from build123d import *

# Parameters (mm, degrees)
SKETCH1_W           = 8
SKETCH1_H           = 16
SKETCH1_R           = 1.55
BOSS_EXTRUDE1_DEPTH = 6
CUT_EXTRUDE1_DEPTH  = 2.5
SKETCH3_W           = 6
SKETCH3_H           = 16
SKETCH3_R           = 0.85
BOSS_EXTRUDE2_DEPTH = 3


with BuildPart() as part:
    # Sketch1 → Boss-Extrude1 (new body)
    with BuildSketch(Plane.XY):
        with Locations((4, 8)):
            Rectangle(SKETCH1_W, SKETCH1_H)
        with Locations((4, 12)):
            Circle(SKETCH1_R, mode=Mode.SUBTRACT)
        with Locations((4, 4)):
            Circle(SKETCH1_R, mode=Mode.SUBTRACT)
    extrude(amount=BOSS_EXTRUDE1_DEPTH)

    # Sketch2 → Cut-Extrude1 (cut)
    with BuildSketch(Plane(origin=(0, 0, 0), x_dir=(-1, 0, 0), z_dir=(0, 0, -1))):
        Polygon((-0.766838493, 12), (-2.383419246, 14.8), (-5.616580754, 14.8), (-7.233161507, 12), (-5.616580754, 9.2), (-2.383419246, 9.2), align=None)
        Polygon((-0.766838493, 4), (-2.383419246, 6.8), (-5.616580754, 6.8), (-7.233161507, 4), (-5.616580754, 1.2), (-2.383419246, 1.2), align=None)
    extrude(amount=-CUT_EXTRUDE1_DEPTH, mode=Mode.SUBTRACT)

    # Sketch3 → Boss-Extrude2 (add)
    # profile 1 of 2: a face of its own
    with BuildSketch(Plane.ZY):
        with Locations((3, 8)):
            Rectangle(SKETCH3_W, SKETCH3_H)
    # profile 2 of 2: a face of its own
    with BuildSketch(Plane.ZY):
        with BuildLine():
            Line((-16.344198667, 10.303286919), (-17.701569131, 12.978645853))
            Line((-17.701569131, 12.978645853), (-24.903097097, 9.324877666))
            ThreePointArc((-24.903097097, 9.324877666), (-20.548417458, 2.41556502), (-12.810955614, -0.198535249))
            Line((-12.810955614, -0.198535249), (0, 0))
            Line((0, 0), (0, 12.465392311))
            Line((0, 12.465392311), (-8.220260468, 12.465392311))
            Line((-8.220260468, 12.465392311), (-9.858504036, 9.95219554))
            ThreePointArc((-9.858504036, 9.95219554), (-13.202702703, 8.255482459), (-16.344198667, 10.303286919))
        make_face()
        with Locations((-13.445945946, 3.76206141)):
            Circle(SKETCH3_R, mode=Mode.SUBTRACT)
        with Locations((-6.088708879, 7.494830187)):
            Circle(SKETCH3_R, mode=Mode.SUBTRACT)
        with Locations((-20.357237067, 8.267231223)):
            Circle(SKETCH3_R, mode=Mode.SUBTRACT)
    extrude(amount=BOSS_EXTRUDE2_DEPTH)


solid = part.part
Read the model definition and answer for the solid it produces. Units are mm, in the model's axes. A direction names the side the tool comes from. Coordinates: 2 decimals unless noted, no trailing zeros. Loops run counter-clockwise (first coordinate to the right, second up) from the corner with the lowest first, then second, coordinate; pieces in that order, holes last. Notation, with made-up numbers: (33, -27) -> (72, -27) arc R25 ccw to (72, -1) -> close; hole circle Ø5 at (22.5, -4.5). An arc over 180 degrees is marked (long way). Answer in a Markdown table with one row per item.
Item 1: A cutting plane is placed at B-B on y = 6. Determine the outline of the cut face in (x, z), plus the area to 3 significant figures.
Returned:
| item | result |
|---|---|
| outline | (-3, -23.62) -> (0, -23.62) -> (0, 0) -> (1.92, 0) -> (1.92, 2.5) -> (6.08, 2.5) -> (6.08, 0) -> (8, 0) -> (8, 6) -> (-3, 6) -> close |
| area | 126 mm^2 |
Item 2: A cutting plane is placed at A-A on x = 4. Determine the outline of the cut face in (y, z).
Returned:
| item | result |
|---|---|
| outline | (0, 0) -> (1.2, 0) -> (1.2, 2.5) -> (2.45, 2.5) -> (2.45, 6) -> (0, 6) -> close; (5.55, 2.5) -> (6.8, 2.5) -> (6.8, 0) -> (9.2, 0) -> (9.2, 2.5) -> (10.45, 2.5) -> (10.45, 6) -> (5.55, 6) -> close; (13.55, 2.5) -> (14.8, 2.5) -> (14.8, 0) -> (16, 0) -> (16, 6) -> (13.55, 6) -> close |
Item 3: A cutting plane is placed at C-C on x = 6.25. Determine the outline of the cut face in (y, z).
Returned:
| item | result |
|---|---|
| outline | (0, 0) -> (2.3, 0) -> (2.3, 2.5) -> (5.7, 2.5) -> (5.7, 0) -> (10.3, 0) -> (10.3, 2.5) -> (13.7, 2.5) -> (13.7, 0) -> (16, 0) -> (16, 6) -> (0, 6) -> close |
Item 4: Each of these flat-tipped pins is pushed along its axis until it touches: P1, Ø3, axis at x = 0.5, z = 4, coming from the -Y side; P2, Ø5, axis at x = 4, y = 12, coming from the -Z side; P3, Ø1.4, axis at y = 3.76, z = -13.45, coming from the -X side; P4, Ø5, axis at y = 2.5, z = -3.5, coming from the +X side. Where does it stop, or does it pass through?
Returned:
| item | result |
|---|---|
| P1 | stops at y = 0 |
| P2 | stops at z = 2.5 |
| P3 | passes through |
| P4 | stops at x = 0 |
Item 5: A cutting plane is placed at D-D on z = -1. Determine the outline of the cut face in (x, y), plus the area to 3 significant figures.
Returned:
| item | result |
|---|---|
| outline | (-3, -0.02) -> (0, -0.02) -> (0, 12.47) -> (-3, 12.47) -> close |
| area | 37.4 mm^2 |
Item 6: Straight lines are drawn through the part: line 1 along Y through (x, z) = (4, 4.7); line 2 along Y through (x, z) = (2.75, 1.5); line 3 along X through (y, z) = (4, 4.2). For each, find the intervals that lie inside material, in ascending order. Write a range as [from, to].
Returned:
| item | result |
|---|---|
| line 1 | y = [0, 2.45], [5.55, 10.45], [13.55, 16] |
| line 2 | y = [0, 1.2], [6.8, 9.2], [14.8, 16] |
| line 3 | x = [-3, 2.45], [5.55, 8] |
Item 7: For faces 1 (the cylindrical face through (-1.479, 7.942, -19.572)), 2 (the cylindrical face through (2.77, 11.06, 4.23)), 3 (the flat face through (6.414, 5.42, 1.232)), 4 (the flat face through (2, 0, 3)), 5 (the flat face through (-1.479, 11.226, -9.028)), determine the directions among +Z, -Z, +X, -X, +Y, -Y from which every point of the face is accessible in a straight line to the end or side of a thin tool.
Returned:
| item | result |
|---|---|
| face 1 | +X, -X |
| face 2 | +Z, -Z |
| face 3 | -Z |
| face 4 | +Z, +X, -X, -Y |
| face 5 | +X, -X, +Y |
Item 8: For a pull along X with two mould halves and no side action, classify faces 6 (the flat face through (-3, 6, -6)), 7 (the flat face through (-1, 12.465, -4)), 8 (the flat face through (1.564, 13.38, 1.232)) as released by +X, released by -X, zero draft, split by the parting line, or undercut.
Returned:
| item | result |
|---|---|
| face 6 | released by -X |
| face 7 | zero draft |
| face 8 | undercut |
